The model under review builds one solid part; all positions refer to its coordinate system, in mm. Face numbers are marked on the shaded views. A direction names the side the tool comes from. Coordinates: 2 decimals unless noted, no trailing zeros. Loops run counter-clockwise (first coordinate to the right, second up) from the corner with the lowest first, then second, coordinate; pieces in that order, holes last. Notation, with made-up numbers: M 73,18 L 125,18 A28 ccw 125,40 Z; hole C 84,55.5 d10. An arc over 180 degrees is marked long. Return JSON: item names as keys, results as strings.
```python
from build123d import *

# Parameters (mm, degrees)
SKETCH1_W           = 27.5
SKETCH1_H           = 19
SKETCH1_W_2         = 22
SKETCH1_H_2         = 12
BOSS_EXTRUDE1_DEPTH = 3.5
SKETCH1_3_W         = 27.5
SKETCH1_3_H         = 4.5
SKETCH1_3_R         = 1
SKETCH1_3_R_2       = 0.5
BOSS_EXTRUDE2_DEPTH = 1
SKETCH1_4_W         = 22
SKETCH1_4_H         = 12
BOSS_EXTRUDE3_DEPTH = 4


with BuildPart() as part:
    # Sketch1 → Boss-Extrude1 (new body)
    with BuildSketch(Plane.XY):
        with Locations((13.75, -10.552238806)):
            Rectangle(SKETCH1_W, SKETCH1_H)
        with Locations((13.75, -8.052238806)):
            Rectangle(SKETCH1_W_2, SKETCH1_H_2, mode=Mode.SUBTRACT)
    extrude(amount=BOSS_EXTRUDE1_DEPTH)

    # Sketch1<3> → Boss-Extrude2 (add)
    # profile 1 of 2: a face of its own
    with BuildSketch(Plane.XY):
        with Locations((13.75, 1.197761194)):
            Rectangle(SKETCH1_3_W, SKETCH1_3_H)
        with Locations((2.5, 0.947761194)):
            Circle(SKETCH1_3_R, mode=Mode.SUBTRACT)
        with Locations((10.75, 1.947761194)):
            Circle(SKETCH1_3_R_2, mode=Mode.SUBTRACT)
        with Locations((12.75, 1.947761194)):
            Circle(SKETCH1_3_R_2, mode=Mode.SUBTRACT)
        with Locations((14.75, 1.947761194)):
            Circle(SKETCH1_3_R_2, mode=Mode.SUBTRACT)
        with Locations((16.75, 1.947761194)):
            Circle(SKETCH1_3_R_2, mode=Mode.SUBTRACT)
        with Locations((25, 0.947761194)):
            Circle(SKETCH1_3_R, mode=Mode.SUBTRACT)
    # profile 2 of 2: a face of its own
    with BuildSketch(Plane.XY):
        with Locations((13.75, -22.302238806)):
            Rectangle(SKETCH1_3_W, SKETCH1_3_H)
        with Locations((2.5, -22.052238806)):
            Circle(SKETCH1_3_R, mode=Mode.SUBTRACT)
        with Locations((25, -22.052238806)):
            Circle(SKETCH1_3_R, mode=Mode.SUBTRACT)
    extrude(amount=BOSS_EXTRUDE2_DEPTH)

    # Sketch1<4> → Boss-Extrude3 (add)
    with BuildSketch(Plane.XY):
        with Locations((13.75, -8.052238806)):
            Rectangle(SKETCH1_4_W, SKETCH1_4_H)
    extrude(amount=BOSS_EXTRUDE3_DEPTH)


solid = part.part
```
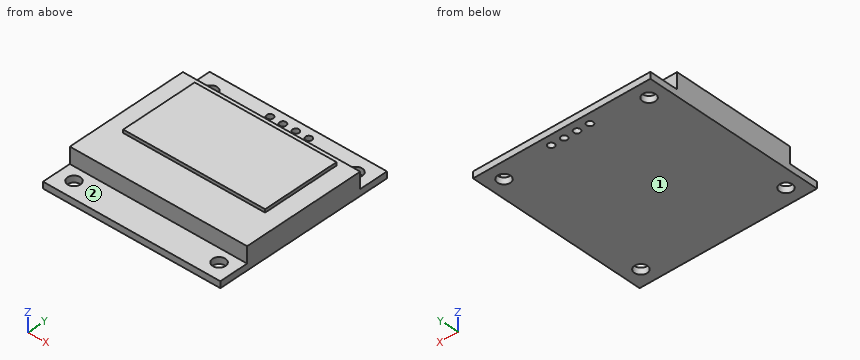
1. Add section D-D on x = 7. Give the boundary of the cut face in (y, z), plus the area to 3 significant figures.
Check values:
{"outline": "M -24.55,0 L 3.45,0 L 3.45,1 L -1.05,1 L -1.05,3.5 L -2.05,3.5 L -2.05,4 L -14.05,4 L -14.05,3.5 L -20.05,3.5 L -20.05,1 L -24.55,1 Z", "area": "81.5 mm²"}
2. Machinability: for the marked faces 1 and 2, which of the approach directions +Z, -Z, +X, -X, +Y, -Y give a long, thin tool a straight path to every point of the face, cutting with its end or side? Answer none if there is none.
Check values:
{"face 1": "-Z, +X, -X, +Y, -Y", "face 2": "+Z, +X, -X, -Y"}
3. Add section C-C on y = -9.25. Give the boundary of the cut face in (x, z).
Check values:
{"outline": "M 0,0 L 27.5,0 L 27.5,3.5 L 24.75,3.5 L 24.75,4 L 2.75,4 L 2.75,3.5 L 0,3.5 Z"}
4. Add section B-B on x = 2. Give the boundary of the cut face in (y, z).
Check values:
{"outline": "M -24.55,0 L -22.92,0 L -22.92,1 L -24.55,1 Z; M -21.19,0 L 0.08,0 L 0.08,1 L -1.05,1 L -1.05,3.5 L -20.05,3.5 L -20.05,1 L -21.19,1 Z; M 1.81,0 L 3.45,0 L 3.45,1 L 1.81,1 Z"}
5. Insertion check: pin 1 Ø2 at (x, z) = (5, 3) entering from +Y; pin 2 Ø1.3 at (x, y) = (14, 0.5) entering from +Z; pin 3 Ø2.5 at (x, y) = (2.5, -22.05) entering from -Z; pin 4 Ø1.2 at (x, z) = (11.5, 2) entering from -Y. Each pin has a flat end and moves straight along its axis. Give the tip position at first contact, or say it passes through.
Check values:
{"pin 1": "y = -1.05", "pin 2": "z = 1", "pin 3": "z = 0", "pin 4": "y = -20.05"}
6. Add section A-A on x = 10.75. Give the boundary of the cut face in (y, z), plus the area to 3 significant figures.
Check values:
{"outline": "M -24.55,0 L 1.45,0 L 1.45,1 L -1.05,1 L -1.05,3.5 L -2.05,3.5 L -2.05,4 L -14.05,4 L -14.05,3.5 L -20.05,3.5 L -20.05,1 L -24.55,1 Z; M 2.45,0 L 3.45,0 L 3.45,1 L 2.45,1 Z", "area": "80.5 mm²"}
7. To check wall thickness, follow line 1 (Y direction, x = 25, z = 0.6); line 2 (Z direction, x = 8.75, y = -21); line 3 (Z direction, x = 4, y = -2). State the ranges of each line that lie inside material, in increasing order.
Check values:
{"line 1": "-24.55 to -23.05, -21.05 to -0.05, 1.95 to 3.45", "line 2": "0 to 1", "line 3": "0 to 3.5"}
